The figure shows three views and two pictorial views of one solid part (mm, origin at its lowest corner). Answer the questions. A direction names the side the tool comes from. Coordinates: 2 decimals unless noted, no trailing zeros. Loops run counter-clockwise (first coordinate to the right, second up) from the corner with the lowest first, then second, coordinate; pieces in that order, holes last.
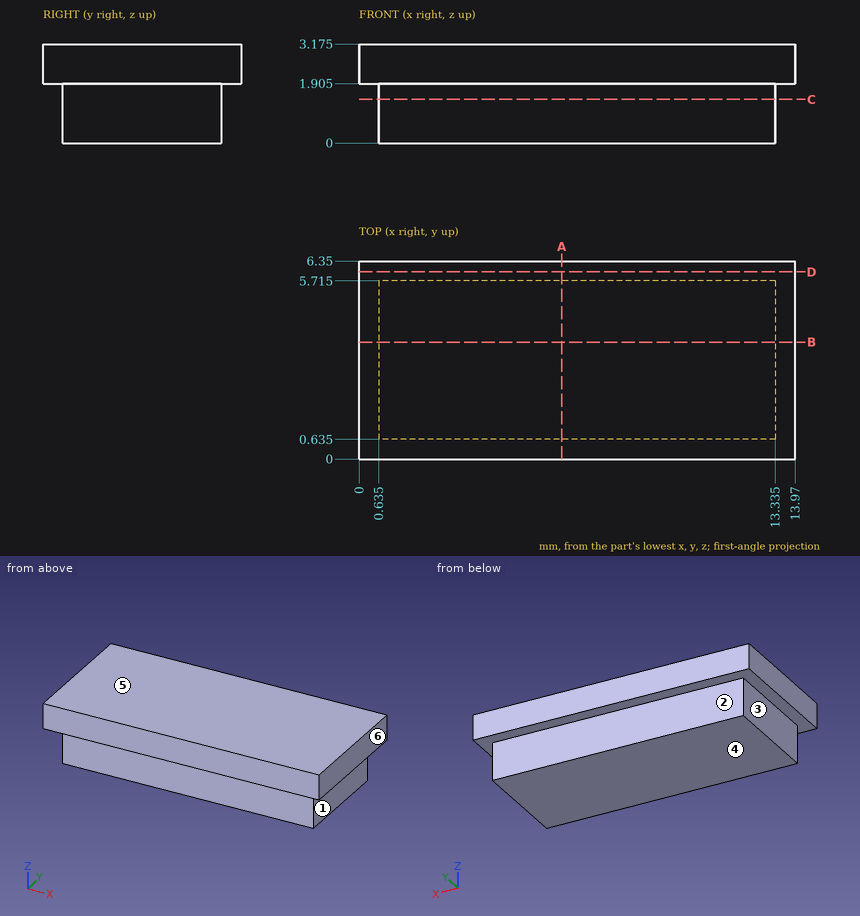
Q1. A cutting plane is placed at D-D (y = 6). Give the vertices of the cut face in (x, z) (3 decimals).
Findings below:
outline: (0, 1.905) - (13.97, 1.905) - (13.97, 3.175) - (0, 3.175) - close
Q2. Which of the six approach directions +Z, -Z, +X, -X, +Y, -Y give full straight-line access (tool end or side, diameter ignored) to the marked faces 1, 2 and 3?
Findings below:
face 1: -Z, +X, +Y, -Y
face 2: -Z, +X, -X, +Y
face 3: -Z, -X, +Y, -Y
Q3. A cutting plane is placed at C-C (z = 1.4). Give the vertices of the cut face in (x, y) (3 decimals), then the cut area to 3 significant figures.
Findings below:
outline: (0.635, 0.635) - (13.335, 0.635) - (13.335, 5.715) - (0.635, 5.715) - close
area: 64.5 mm2
Q4. Flat-ended cylindrical pins translate along their axes: pin 1 Ø1.5 at (y, z) = (3, 1.5) entering from +X; pin 2 Ø0.6 at (x, z) = (4, 1) entering from +Y (3 decimals); pin 3 Ø0.6 at (y, z) = (3, 1.5) entering from -X (3 decimals). Find the tip coordinate at first contact, or state that the pin passes through.
Findings below:
pin 1: stops at x = 13.97
pin 2: stops at y = 5.715
pin 3: stops at x = 0.635
Q5. Determine the mould class of the marked faces 4, 5 and 6 for opening direction Z: +Z half, -Z half, draft (parallel to the pull), parting line (faces both ways), or undercut.
Findings below:
face 4: -Z half
face 5: +Z half
face 6: draft
Q6. A cutting plane is placed at B-B (y = 3.75). Give the vertices of the cut face in (x, z) (3 decimals).
Findings below:
outline: (0, 1.905) - (0.635, 1.905) - (0.635, 0) - (13.335, 0) - (13.335, 1.905) - (13.97, 1.905) - (13.97, 3.175) - (0, 3.175) - close
Q7. Straight lines are drawn through the part: probe 1 along Y at (x, z) = (6, 0.9) (3 decimals); probe 2 along Z at (x, y) = (1, 0.5) (3 decimals); probe 3 along X at (y, z) = (1, 0.95) (3 decimals). For each, find the intervals that lie inside material, in ascending order.
Findings below:
probe 1: y = 0.635 to 5.715
probe 2: z = 1.905 to 3.175
probe 3: x = 0.635 to 13.335
Q8. A cutting plane is placed at A-A (x = 6.5). Give the vertices of the cut face in (y, z) (3 decimals), then the cut area to 3 significant figures.
Findings below:
outline: (0, 1.905) - (0.635, 1.905) - (0.635, 0) - (5.715, 0) - (5.715, 1.905) - (6.35, 1.905) - (6.35, 3.175) - (0, 3.175) - close
area: 17.7 mm2
